Build history of the part. All positions in model axes, mm. A direction names the side the tool comes from. Give positions to 0.01 mm unless a question says otherwise; leave off trailing zeros. Order: outer loops, then holes, each group sorted by start corner. A loop starts at its lowest first (then second) coordinate and runs counter-clockwise, first axis right, second up. Notation, with made-up numbers: M 25,87.5 L 54,87.5 A12 ccw 54,100.5 Z; hole C 77,51.5 d9. An arc over 180 degrees is marked long. Use CSV: the item, a comma, the result in double quotes. Start each with the question number.
Item 1: Band-saw the part on B-B on y = 13.5. Write the cut outline in (x, z).
Item 2: Band-saw the part on A-A on z = 12. Write the cut outline in (x, y), plus the area to 3 significant figures.
Item 3: Two-plate mould, pull along X, no slides. Class faces 4 (the flat face through (15, 20, 15)), 5 (the flat face through (-10, 11, 15)), 6 (the flat face through (20, 10, 15)): pulls with the +X half, pulls with the -X half, needs draft (parallel to the pull), parting line crosses it, or undercut.
Item 4: Band-saw the part on C-C on z = 25.5. Write the cut outline in (x, y), plus the area to 3 significant figures.
Item 5: Pin check, flat tips, straight feed: P1, Ø1.5, axis at x = 7, z = 8, coming from the +Y side; P2, Ø5, axis at y = 14, z = 6, coming from the +X side. Stop position of each tip, or through.
Item 6: Which spindle directions (+Z, -Z, +X, -X, +Y, -Y) get a long thin tool onto all of the face, cutting with end or side? Do faces 1 (the flat face through (10, 11, 15)), 2 (the cylindrical face through (-14.93, 10.583, 6.759)), 3 (the cylindrical face through (-14.93, 18.289, 28.196)). Say none if no direction does.
Item 7: Wall check: line 1 along Z through (x, y) = (17.5, 14); line 2 along Y through (x, z) = (13.25, 6); line 3 along X through (y, z) = (15, 11.5). Give the ranges that are in metal, low to high.
Item 8: Band-saw the part on D-D on x = 2. Write the cut outline in (y, z).
from build123d import *

# Parameters (mm, degrees)
BOSS_EXTRUDE1_DEPTH = 30
FILLET1_R           = 6
SKETCH2_R           = 3.5
CUT_EXTRUDE1_DEPTH  = 30
SKETCH3_R           = 2.75
CUT_EXTRUDE2_DEPTH  = 30


with BuildPart() as part:
    # Sketch1 → Boss-Extrude1 (new body)
    with BuildSketch(Plane.XY):
        Polygon((0, 0), (-20, 0), (-20, 20), (-10, 20), (-10, 2), (10, 2), (10, 20), (20, 20), (20, 0), align=None)
    extrude(amount=BOSS_EXTRUDE1_DEPTH)

    # Fillet1
    fillet1_edges = [part.edges().sort_by_distance(p)[0] for p in [
        (15, 20, 30),
        (15, 20, 0),
        (-15, 20, 30),
        (-15, 20, 0),
    ]]
    fillet(fillet1_edges, radius=FILLET1_R)

    # Sketch2 → Cut-Extrude1 (cut)
    with BuildSketch(Plane(origin=(0, 0, 0), x_dir=(0, 0, -1), z_dir=(1, 0, 0))):
        with Locations((-24, 14)):
            Circle(SKETCH2_R)
        with Locations((-6, 14)):
            Circle(SKETCH2_R)
    extrude(amount=-CUT_EXTRUDE1_DEPTH, mode=Mode.SUBTRACT)

    # Sketch3 → Cut-Extrude2 (cut)
    with BuildSketch(Plane(origin=(0, 0, 0), x_dir=(0, 0, -1), z_dir=(1, 0, 0))):
        with Locations(Location((-6, 14, 0), (0, 0, 90))):
            Circle(SKETCH3_R)
        with Locations(Location((-24, 14, 0), (0, 0, 90))):
            Circle(SKETCH3_R)
    extrude(amount=CUT_EXTRUDE2_DEPTH, mode=Mode.SUBTRACT)


solid = part.part
Model answer:
1,outline,"M -20,0 L -10,0 L -10,2.54 L -20,2.54 Z; M -20,9.46 L -10,9.46 L -10,20.54 L -20,20.54 Z; M -20,27.46 L -10,27.46 L -10,30 L -20,30 Z; M 10,0 L 20,0 L 20,3.3 L 10,3.3 Z; M 10,8.7 L 20,8.7 L 20,21.3 L 10,21.3 Z; M 10,26.7 L 20,26.7 L 20,30 L 10,30 Z"
2,outline,"M -20,0 L 20,0 L 20,20 L 10,20 L 10,2 L -10,2 L -10,20 L -20,20 Z"
2,area,"440 mm^2"
3,face 4,"needs draft"
3,face 5,"undercut"
3,face 6,"pulls with the +X half"
4,outline,"M -20,0 L 20,0 L 20,11.7 L 10,11.7 L 10,2 L -10,2 L -10,10.84 L -20,10.84 Z; M -20,17.16 L -10,17.16 L -10,19.81 L -20,19.81 Z; M 10,16.3 L 20,16.3 L 20,19.81 L 10,19.81 Z"
4,area,"327 mm^2"
5,P1,"stops at y = 2"
5,P2,"passes through"
6,face 1,"+Z, -Z, +Y"
6,face 2,"-X"
6,face 3,"+Z, +X, -X, +Y"
7,line 1,"z = 0 to 3.25, 8.75 to 21.25, 26.75 to 30"
7,line 2,"y = 0 to 11.25, 16.75 to 20"
7,line 3,"x = -20 to -10, 10 to 20"
8,outline,"M 0,0 L 2,0 L 2,30 L 0,30 Z"
